from build123d import *

# Parameters (mm, degrees)
SKETCH1_W                = 30
SKETCH1_H                = 30
BOSS_EXTRUDE1_DEPTH      = 41
SKETCH2_R                = 3.375
CUT_EXTRUDE1_DEPTH       = 83
FILLET1_R                = 2.5
CUT_EXTRUDE2_DEPTH       = 83
CIRPATTERN1_COUNT        = 4
CIRPATTERN1_COPY_1_DEPTH = 83
CIRPATTERN1_COPY_2_DEPTH = 83
CIRPATTERN1_COPY_3_DEPTH = 83


with BuildPart() as part:
    # Sketch1 → Boss-Extrude1 (new body, symmetric)
    with BuildSketch(Plane.XY):
        Rectangle(SKETCH1_W, SKETCH1_H)
    extrude(amount=BOSS_EXTRUDE1_DEPTH, both=True)

    # Sketch2 → Cut-Extrude1 (cut, through all)
    with BuildSketch(Plane.XY.offset(41)):
        Circle(SKETCH2_R)
    extrude(amount=-CUT_EXTRUDE1_DEPTH, mode=Mode.SUBTRACT)

    # Fillet1
    fillet1_edges = [part.edges().sort_by_distance(p)[0] for p in [
        (15, -15, 0),
        (-15, -15, 0),
        (-15, 15, 0),
        (15, 15, 0),
    ]]
    fillet(fillet1_edges, radius=FILLET1_R)

    # Sketch3 → Cut-Extrude2 (cut, through all)
    with BuildSketch(Plane.XY.offset(41)):
        Polygon((0, 15), (-5.1, 15), (-5.1, 14.2), (-4.25, 14.2), (-4.25, 13.2), (-8.375, 13.2), (-8.375, 9.9), (-5.975, 7.5), (0, 7.5), align=None)
    cut_extrude2 = extrude(amount=-CUT_EXTRUDE2_DEPTH, mode=Mode.SUBTRACT)

    # Mirror1: Cut-Extrude2 across plane
    add(cut_extrude2.mirror(Plane(origin=(0, 0, 0), x_dir=(0, 0, 1), z_dir=(1, 0, 0))), mode=Mode.SUBTRACT)

    # CirPattern1: Cut-Extrude2 ×4 about axis
    cirpattern1_axis = Axis((0, 0, 0), (0, 0, 1))
    for i in range(1, CIRPATTERN1_COUNT):
        add(cut_extrude2.rotate(cirpattern1_axis, i * 360 / CIRPATTERN1_COUNT), mode=Mode.SUBTRACT)

    # CirPattern1 copy 1 sketch → CirPattern1 copy 1 (cut, through all)
    with BuildSketch(Plane(origin=(0, 0, 41), x_dir=(0, -1, 0), z_dir=(0, 0, 1))):
        Polygon((0, -15), (-5.1, -15), (-5.1, -14.2), (-4.25, -14.2), (-4.25, -13.2), (-8.375, -13.2), (-8.375, -9.9), (-5.975, -7.5), (0, -7.5), align=None)
    extrude(amount=-CIRPATTERN1_COPY_1_DEPTH, mode=Mode.SUBTRACT)

    # CirPattern1 copy 2 sketch → CirPattern1 copy 2 (cut, through all)
    with BuildSketch(Plane.XY.offset(41)):
        Polygon((0, -15), (-5.1, -15), (-5.1, -14.2), (-4.25, -14.2), (-4.25, -13.2), (-8.375, -13.2), (-8.375, -9.9), (-5.975, -7.5), (0, -7.5), align=None)
    extrude(amount=-CIRPATTERN1_COPY_2_DEPTH, mode=Mode.SUBTRACT)

    # CirPattern1 copy 3 sketch → CirPattern1 copy 3 (cut, through all)
    with BuildSketch(Plane(origin=(0, 0, 41), x_dir=(0, 1, 0), z_dir=(0, 0, 1))):
        Polygon((0, -15), (-5.1, -15), (-5.1, -14.2), (-4.25, -14.2), (-4.25, -13.2), (-8.375, -13.2), (-8.375, -9.9), (-5.975, -7.5), (0, -7.5), align=None)
    extrude(amount=-CIRPATTERN1_COPY_3_DEPTH, mode=Mode.SUBTRACT)


solid = part.part
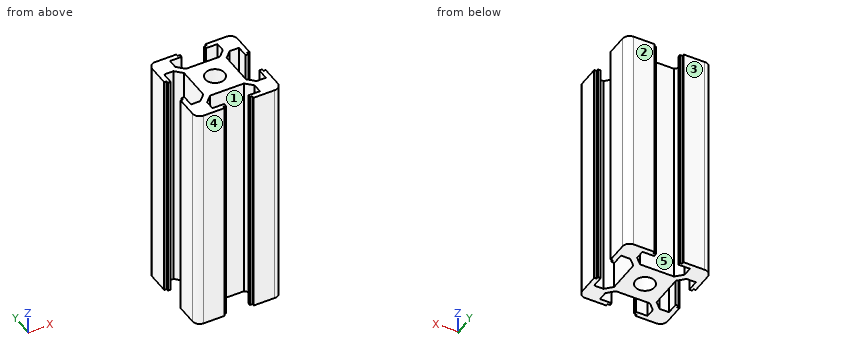
Can you work these out from the model? Positions are in its coordinate system, mm. Face numbers are marked on the shaded views. A direction names the side the tool comes from. Coordinates: 2 decimals unless noted, no trailing zeros. Write each loop counter-clockwise with the first axis right and the second up, starting at its lowest first coordinate (ties: lowest second). Pieces come first, ordered by that corner, then holes. Notation, with made-up numbers: (52, -26.5) -> (70, -26.5) arc R12 cw to (70, -18.5) -> close; hole circle Ø3 at (1.5, 50). An arc over 180 degrees is marked (long way). Write each question's results on one line, items separated by ' | '. Start each with the question number.
Q1. Imagine slicing it at A-A (x = 0). Write out the boundary of the cut face in (y, z) (3 decimals).
Q2. I'm going to push flat-ended pins straight in: pin 1 (1.1 mm diameter, centred on y = -13.5, z = 12.5, fed in from +X); pin 2 (5 mm diameter, centred on x = -2, z = 30.5, fed in from +Y); pin 3 (0.8 mm diameter, centred on x = -13.5, z = 15.5, fed in from +Y). Where does each tip first touch, or does it pass through?
Q3. We'd pull the mould along Y, two halves only. Please class the marked faces 3, 4 and 5: +Y half, -Y half, draft (parallel to the pull), parting line (faces both ways), or undercut.
Q4. If I drill on probe 1 along Y at (x, z) = (0, -22) (3 decimals); probe 2 along X at (y, z) = (-10.25, -34) (3 decimals); probe 3 along Y at (x, z) = (4.5, 25), over which ranges is the centre line in solid material (lowest first)?
Q5. On a 3-axis mill with a long thin cutter (end or side, diameter ignored), from which of +Z, -Z, +X, -X, +Y, -Y can I reach the whole of each face in a straight line? I mean the marked faces 1 and 2. Say none if no direction works.
Taken from the geometry:
1) outline: (-7.5, -41) -> (-3.375, -41) -> (-3.375, 41) -> (-7.5, 41) -> close; (3.375, -41) -> (7.5, -41) -> (7.5, 41) -> (3.375, 41) -> close
2) pin 1: stops at x = 14.96 | pin 2: stops at y = 14.2 | pin 3: stops at y = 14.93
3) face 3: +Y half | face 4: -Y half | face 5: undercut
4) probe 1: y = -7.5 to -3.375, 3.375 to 7.5 | probe 2: x = -15 to -8.375, 8.375 to 15 | probe 3: y = -14.2 to -13.2, -7.5 to 7.5, 13.2 to 14.2
5) face 1: +Z, -Z | face 2: +Z, -Z, +X, -X, +Y
